Can you work these out from the model? Positions are in its coordinate system, mm. Give positions to 0.01 mm unless a question says otherwise; leave off trailing zeros. Order: outer loops, then holes, each group sorted by start corner. A loop starts at its lowest first (then second) coordinate and runs counter-clockwise, first axis right, second up. Notation, with made-up numbers: (44.5, 11) -> (48.5, 11) arc R16 ccw to (48.5, 32) -> close; hole circle Ø1 at (74.5, 17.5). An arc over 180 degrees is marked (long way). Answer as a JSON object with one key per item and string values.
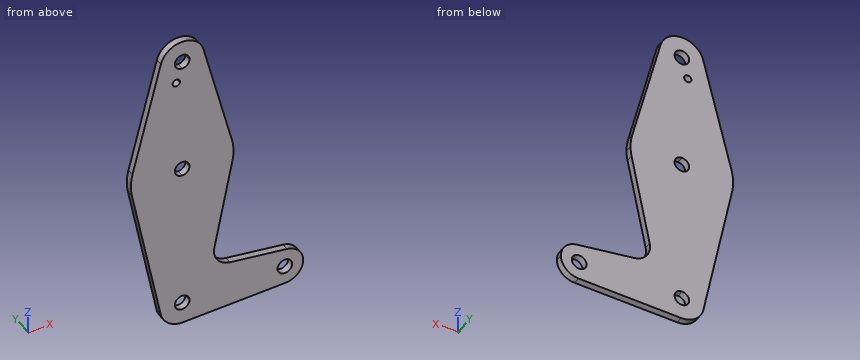
```python
from build123d import *

# Parameters (mm, degrees)
F0_R     = 3.175
F1_DEPTH = 3.048


with BuildPart() as f1:
    # F0 (on Front) → F1 (new body)
    with BuildSketch(Plane.XZ):
        with BuildLine():
            ThreePointArc((-1.0023336327, 43.4057982907), (-0.5018639238, 43.3661433225), (0, 43.3529127479))
            ThreePointArc((0, 43.3529127479), (6.7351920908, 46.1427206571), (9.525, 52.8779127479))
            ThreePointArc((9.525, 52.8779127479), (9.4490828569, 54.0781036338), (9.2225415932, 55.2591627479))
            ThreePointArc((9.2225415932, 55.2591627479), (0, 62.4029127479), (-9.2225415932, 55.2591627479))
            ThreePointArc((-9.2225415932, 55.2591627479), (-8.6217427785, 48.8293109569), (-4.0577774611, 44.2604846468))
            ThreePointArc((-4.0577774611, 44.2604846468), (-2.3007024801, 45.3437609387), (-0.9587182239, 43.7753610313))
            ThreePointArc((-0.9587182239, 43.7753610313), (-0.9696597824, 43.5892972498), (-1.0023336327, 43.4057982907))
        make_face()
        with BuildLine():
            ThreePointArc((3.175, 52.8779127479), (2.2450640303, 50.6328487176), (0, 49.7029127479))
            ThreePointArc((0, 49.7029127479), (-2.2450640303, 55.1229767781), (3.175, 52.8779127479))
        make_face(mode=Mode.SUBTRACT)
        with BuildLine():
            ThreePointArc((9.525, 52.8779127479), (6.7351920908, 46.1427206571), (0, 43.3529127479))
            Line((0, 43.3529127479), (0, 24.3029127479))
            ThreePointArc((0, 24.3029127479), (13.6099773833, 19.6483179972), (21.5192637174, 7.6341627479))
            Line((21.5192637174, 7.6341627479), (9.2225415932, 55.2591627479))
            ThreePointArc((9.2225415932, 55.2591627479), (9.4490828569, 54.0781036338), (9.525, 52.8779127479))
        make_face()
        with BuildLine():
            Line((0, 24.3029127479), (0, 43.3529127479))
            ThreePointArc((0, 43.3529127479), (-0.5018639238, 43.3661433225), (-1.0023336327, 43.4057982907))
            ThreePointArc((-1.0023336327, 43.4057982907), (-2.9738669395, 42.2465468418), (-4.0577774611, 44.2604846468))
            ThreePointArc((-4.0577774611, 44.2604846468), (-8.6217427785, 48.8293109569), (-9.2225415932, 55.2591627479))
            Line((-9.2225415932, 55.2591627479), (-21.5192637174, 7.6341627479))
            ThreePointArc((-21.5192637174, 7.6341627479), (-13.6099773833, 19.6483179972), (0, 24.3029127479))
        make_face()
        with BuildLine():
            ThreePointArc((21.5192637174, 7.6341627479), (13.6099773833, 19.6483179972), (0, 24.3029127479))
            Line((0, 24.3029127479), (0, 5.2529127479))
            ThreePointArc((0, 5.2529127479), (2.2450640303, 4.3229767781), (3.175, 2.0779127479))
            ThreePointArc((3.175, 2.0779127479), (2.2450640303, -0.1671512824), (0, -1.0970872521))
            Line((0, -1.0970872521), (0, -20.1470872521))
            ThreePointArc((0, -20.1470872521), (14.0563241994, -15.137498226), (21.7759638133, -2.3670872521))
            ThreePointArc((21.7759638133, -2.3670872521), (22.1124560005, -0.1558989327), (22.225, 2.0779127479))
            ThreePointArc((22.225, 2.0779127479), (22.0478599995, 4.8783581483), (21.5192637174, 7.6341627479))
        make_face()
        with BuildLine():
            Line((0, 5.2529127479), (0, 24.3029127479))
            ThreePointArc((0, 24.3029127479), (-13.6099773833, 19.6483179972), (-21.5192637174, 7.6341627479))
            ThreePointArc((-21.5192637174, 7.6341627479), (-22.2176828703, 2.6481695983), (-21.7759638133, -2.3670872521))
            ThreePointArc((-21.7759638133, -2.3670872521), (-14.0563241994, -15.137498226), (0, -20.1470872521))
            Line((0, -20.1470872521), (0, -1.0970872521))
            ThreePointArc((0, -1.0970872521), (-3.175, 2.0779127479), (0, 5.2529127479))
        make_face()
        with BuildLine():
            ThreePointArc((0, -20.1470872521), (-14.0563241994, -15.137498226), (-21.7759638133, -2.3670872521))
            Line((-21.7759638133, -2.3670872521), (-9.33255592, -63.3270872521))
            ThreePointArc((-9.33255592, -63.3270872521), (-7.3780332745, -55.3979483095), (0, -51.8970872521))
            Line((0, -51.8970872521), (0, -20.1470872521))
        make_face()
        with BuildLine():
            ThreePointArc((21.7759638133, -2.3670872521), (14.0563241994, -15.137498226), (0, -20.1470872521))
            Line((0, -20.1470872521), (0, -51.8970872521))
            ThreePointArc((0, -51.8970872521), (6.7351920908, -54.6868951613), (9.525, -61.4220872521))
            ThreePointArc((9.525, -61.4220872521), (6.8544083402, -68.0359145334), (0.3401787284, -70.9410106909))
            Line((0.3401787284, -70.9410106909), (44.7334821429, -69.3545234558))
            ThreePointArc((44.7334821429, -69.3545234558), (36.5213147589, -61.0481131928), (45.4788644675, -53.5515507928))
            Line((45.4788644675, -53.5515507928), (20.682408707, -50.3100700647))
            ThreePointArc((20.682408707, -50.3100700647), (15.241157261, -47.0445132049), (13.9233460165, -40.836900747))
            Line((13.9233460165, -40.836900747), (21.7759638133, -2.3670872521))
        make_face()
        with BuildLine():
            ThreePointArc((0, -51.8970872521), (-7.3780332745, -55.3979483095), (-9.33255592, -63.3270872521))
            ThreePointArc((-9.33255592, -63.3270872521), (-5.8914064044, -68.9065348322), (0.3401787284, -70.9410106909))
            ThreePointArc((0.3401787284, -70.9410106909), (6.8544083402, -68.0359145334), (9.525, -61.4220872521))
            ThreePointArc((9.525, -61.4220872521), (6.7351920908, -54.6868951613), (0, -51.8970872521))
        make_face()
        with BuildLine():
            ThreePointArc((3.175, -61.4220872521), (-2.2450640303, -63.6671512824), (0, -58.2470872521))
            ThreePointArc((0, -58.2470872521), (2.2450640303, -59.1770232219), (3.175, -61.4220872521))
        make_face(mode=Mode.SUBTRACT)
        with BuildLine():
            ThreePointArc((45.4788644675, -53.5515507928), (36.5213147589, -61.0481131928), (44.7334821429, -69.3545234558))
            ThreePointArc((44.7334821429, -69.3545234558), (50.1620069047, -66.9336100336), (52.3875, -61.4220872521))
            ThreePointArc((52.3875, -61.4220872521), (50.4153381279, -56.1858054349), (45.4788644675, -53.5515507928))
        make_face()
        with Locations((44.45, -61.4220872521)):
            Circle(F0_R, mode=Mode.SUBTRACT)
    extrude(amount=F1_DEPTH)


solid = f1.part
```
1. If we section it at A-A on x = 38: Please give me the cut outline in (y, z), then the cut area to 3 significant figures.
Worked answers:
{"outline": "(-3.05, -69.6) -> (0, -69.6) -> (0, -52.57) -> (-3.05, -52.57) -> close", "area": "51.9 mm²"}
2. Please list where these lines run through material, in increasing order: L1, parallel to Z at x = 2.5, y = -2.65; L2, parallel to X at y = -2.7, z = -61; L3, parallel to X at y = -2.4, z = -58.5.
Worked answers:
{"L1": "-70.86 to -63.38, -59.46 to 0.12, 4.04 to 50.92, 54.84 to 62.07", "L2": "-9.81 to -3.15, 3.15 to 41.3, 47.6 to 52.38", "L3": "-10.32 to -1.24, 1.24 to 43.21, 45.69 to 51.83"}
3. If we section it at B-B on z = -27: Please give me the cut outline in (x, y).
Worked answers:
{"outline": "(-16.75, -3.05) -> (16.75, -3.05) -> (16.75, 0) -> (-16.75, 0) -> close"}
4. Will this pin go through, and if not, where does the flat tip stop? pin 1 Ø1.5 at (x, y) = (-6, -1) entering from +Z.
Worked answers:
{"pin 1": "z = 60.83"}
